```python
from build123d import *

# Parameters (mm, degrees)
BOSS_EXTRUDE1_DEPTH = 156.99994
SKETCH2_R           = 2
CUT_EXTRUDE1_DEPTH  = 16


with BuildPart() as part:
    # Sketch1 → Boss-Extrude1 (new body)
    with BuildSketch(Plane.XY):
        with BuildLine():
            Line((-6.5, 0), (6.5, 0))
            Line((6.5, 0), (6.5, 5.2))
            Line((6.5, 5.2), (4.8, 6.9))
            Line((4.8, 6.9), (4.8, 8.84))
            Line((4.8, 8.84), (5.754868434, 9.794868434))
            ThreePointArc((5.754868434, 9.794868434), (6.196913421, 10.683086579), (7.085131566, 11.125131566))
            Line((7.085131566, 11.125131566), (7.5, 11.54))
            Line((7.5, 11.54), (7.5, 12.85))
            Line((7.5, 12.85), (7.08164233, 13.26835767))
            ThreePointArc((7.08164233, 13.26835767), (6.196913421, 13.709913421), (5.75535767, 14.59464233))
            Line((5.75535767, 14.59464233), (5.35, 15))
            Line((5.35, 15), (-5.35, 15))
            Line((-5.35, 15), (-5.75535767, 14.59464233))
            ThreePointArc((-5.75535767, 14.59464233), (-6.196913421, 13.709913421), (-7.08164233, 13.26835767))
            Line((-7.08164233, 13.26835767), (-7.5, 12.85))
            Line((-7.5, 12.85), (-7.5, 11.54))
            Line((-7.5, 11.54), (-7.085131566, 11.125131566))
            ThreePointArc((-7.085131566, 11.125131566), (-6.196913421, 10.683086579), (-5.754868434, 9.794868434))
            Line((-5.754868434, 9.794868434), (-4.8, 8.84))
            Line((-4.8, 8.84), (-4.8, 6.9))
            Line((-4.8, 6.9), (-6.5, 5.2))
            Line((-6.5, 5.2), (-6.5, 0))
        make_face()
    extrude(amount=BOSS_EXTRUDE1_DEPTH)

    # Sketch2 → Cut-Extrude1 (cut, through all)
    with BuildSketch(Plane(origin=(0, 15, 0), x_dir=(1, 0, 0), z_dir=(0, 1, 0))):
        with Locations((0, -20)):
            Circle(SKETCH2_R)
        with Locations((0, -79.944)):
            Circle(SKETCH2_R)
        with Locations((0, -139.888)):
            Circle(SKETCH2_R)
    extrude(amount=-CUT_EXTRUDE1_DEPTH, mode=Mode.SUBTRACT)


solid = part.part
```
Work out the finished part from the listing and answer in its coordinate system (mm). A direction names the side the tool comes from. Give positions to 0.01 mm unless a question says otherwise; leave off trailing zeros. Loops run counter-clockwise (first coordinate to the right, second up) from the corner with the lowest first, then second, coordinate; pieces in that order, holes last. Notation, with made-up numbers: (-7, 75.25) -> (52, 75.25) arc R26 ccw to (52, 114.25) -> close; hole circle Ø11 at (69, -2.5). An arc over 180 degrees is marked (long way). Put each result on its own line as item: value. Start each with the question number.
Item 1: The part is cut by section A-A (z = 20). Give the vertices of the cut face in (x, y).
Item 2: The part is cut by section B-B (x = 0). Give the vertices of the cut face in (y, z).
Item 3: Each of these flat-tipped pins is pushed along its axis until it touches: P1, Ø4, axis at y = 3.5, z = 57.5, coming from the +X side; P2, Ø2.5, axis at y = 3, z = 104.5, coming from the -X side; P3, Ø2, axis at y = 8, z = 93, coming from the +X side. Where does it stop, or does it pass through?
Item 4: Find the intervals of material crossed by L1, parallel to Z at x = 0, y = 3.5; L2, parallel to Y at x = 5, z = 46; L3, parallel to X at y = 10, z = 20, in increasing order. Write a range as [from, to].
Item 5: Which of the six approach directions +Z, -Z, +X, -X, +Y, -Y give full straight-line access (tool end or side, diameter ignored) to faces 1 (the face through (-6.5, 3, 77)), 2 (the face through (0, 0, 77))?
Item 6: The mould has two halves that part along X. Classify faces 3 (the face through (0, 8, 0)), 4 (the face through (0, 8, 18)), 5 (the face through (6.5, 3, 77)), 6 (the face through (0.923, 7.605, 141.662)): released by +X, released by -X, zero draft, split by the parting line, or undercut.
Answers below:
1. outline: (-7.5, 11.54) -> (-7.09, 11.13) arc R1.56 cw to (-5.75, 9.79) -> (-4.8, 8.84) -> (-4.8, 6.9) -> (-6.5, 5.2) -> (-6.5, 0) -> (-2, 0) -> (-2, 15) -> (-5.35, 15) -> (-5.76, 14.59) arc R1.56 cw to (-7.08, 13.27) -> (-7.5, 12.85) -> close; (2, 0) -> (6.5, 0) -> (6.5, 5.2) -> (4.8, 6.9) -> (4.8, 8.84) -> (5.75, 9.79) arc R1.56 cw to (7.09, 11.13) -> (7.5, 11.54) -> (7.5, 12.85) -> (7.08, 13.27) arc R1.56 cw to (5.76, 14.59) -> (5.35, 15) -> (2, 15) -> close
2. outline: (0, 0) -> (15, 0) -> (15, 18) -> (0, 18) -> close; (0, 22) -> (15, 22) -> (15, 77.94) -> (0, 77.94) -> close; (0, 81.94) -> (15, 81.94) -> (15, 137.89) -> (0, 137.89) -> close; (0, 141.89) -> (15, 141.89) -> (15, 157) -> (0, 157) -> close
3. P1: x = 6.5
3. P2: x = -6.5
3. P3: x = 4.96
4. L1: [0, 18], [22, 77.94], [81.94, 137.89], [141.89, 157]
4. L2: [0, 6.7], [9.04, 15]
4. L3: [-5.8, -2], [2, 5.8]
5. face 1: +Z, -Z, -X, -Y
5. face 2: +Z, -Z, +X, -X, -Y
6. face 3: zero draft
6. face 4: undercut
6. face 5: released by +X
6. face 6: undercut
